Design review of the part shown in the three views and the two pictorial views. Dimensions are in mm from the part's minimum x, y and z. Round coordinates to 2 decimals unless told otherwise and drop trailing zeros. Write each loop counter-clockwise with the first axis right and the second up, starting at its lowest first coordinate (ties: lowest second). Pieces come first, ordered by that corner, then holes. Notation, with made-up numbers: (4.5, -23) - (47.5, -23) arc R17 ccw to (47.5, -4) - close; hole circle Ø4 at (-24, 81.25). An arc over 180 degrees is marked (long way). Use one line per item in the form item = value.
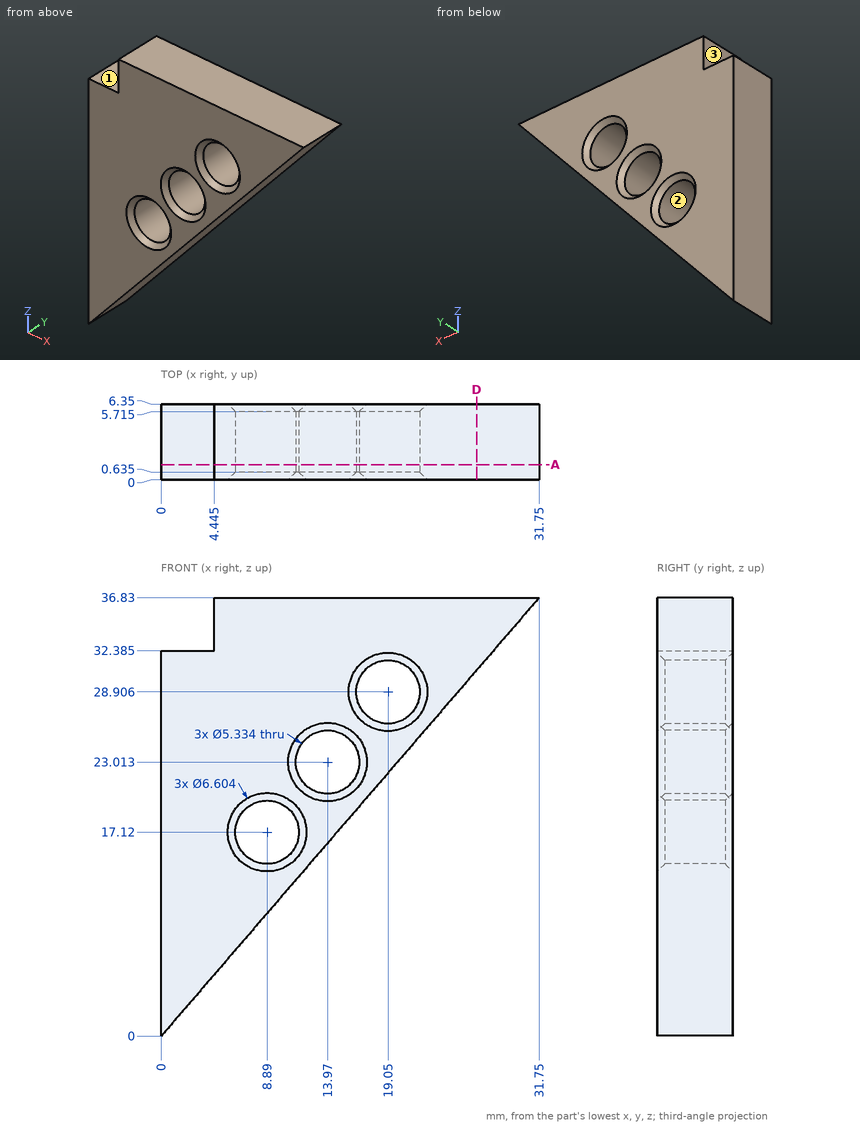
(1) Add section A-A on y = 1.25. Count the separate pieces of the cut face and the enclosed holes in it, then the cut area to 3 significant figures.
Geometry results:
separate_pieces = 1
enclosed_holes = 3
area = 498 mm2
(2) To check wall thickness, follow L1, parallel to Z at x = 10, y = 1 (1 decimal); L2, parallel to X at y = 1.25, z = 19; L3, parallel to Z at x = 11, y = 3.75. State the ranges of each line that lie inside material, in increasing order.
Geometry results:
L1 = 11.6 to 14.7, 19.5 to 36.8
L2 = 0 to 7, 10.78 to 16.38
L3 = 12.76 to 15.49, 18.75 to 36.83
(3) The part is to be moulded in two halves that separate along Z. For the marked faces 1, 2 and 3, say which applies: +Z half, -Z half, draft (parallel to the pull), parting line (faces both ways), or undercut.
Geometry results:
face_1 = +Z half
face_2 = undercut
face_3 = draft
(4) Insertion check: P1, Ø1.5, axis at x = 4, y = 2, coming from the +Z side; P2, Ø3.5, axis at x = 1.5, y = 2.5, coming from the +Z side (3 decimals); P3, Ø3.5, axis at y = 2.5, z = 34.5, coming from the -X side (3 decimals); P4, Ø6, axis at x = 19.05, z = 28.91, coming from the -Y side. Each pin has a flat end and moves straight along its axis. Give the tip position at first contact, or say it passes through.
Geometry results:
P1 = 36.83
P2 = 32.385
P3 = 4.445
P4 = 0.3
(5) Add section D-D on x = 26.5. Write out the cut boundary in (y, z).
Geometry results:
outline = (0, 30.74) - (6.35, 30.74) - (6.35, 36.83) - (0, 36.83) - close
